from build123d import *

# Parameters (mm, degrees)
BOSS_EXTRUDE1_DEPTH = 6.35
SKETCH2_W           = 6.35
SKETCH2_H           = 1.5875
CUT_EXTRUDE1_DEPTH  = 6.35
BOSS_EXTRUDE2_START = -6.35
SKETCH4_W           = 24.326613467
SKETCH4_H           = 69.85
BOSS_EXTRUDE2_DEPTH = 6.35
SKETCH5_W           = 25.4
SKETCH5_H           = 3.175
CUT_EXTRUDE3_DEPTH  = 6.35
SKETCH7_W           = 19.923596682
SKETCH7_H           = 95.25
CUT_EXTRUDE4_DEPTH  = 6.35
SKETCH8_W           = 15.043251586
SKETCH8_H           = 69.85
CUT_EXTRUDE5_DEPTH  = 6.35
SKETCH9_W           = 3.175
SKETCH9_H           = 95.25
BOSS_EXTRUDE3_DEPTH = 6.35
SKETCH10_W          = 17.539756693
SKETCH10_H          = 95.25
CUT_EXTRUDE7_DEPTH  = 6.35
SKETCH3_W           = 4.7625
SKETCH3_H           = 14.2875
SKETCH3_W_2         = 9.525
SKETCH3_H_2         = 3.175
CUT_EXTRUDE8_DEPTH  = 6.35
SKETCH11_W          = 14.2875
SKETCH11_H          = 4.7625
SKETCH11_W_2        = 3.175
SKETCH11_H_2        = 7.9375
CUT_EXTRUDE9_DEPTH  = 6.35
SKETCH14_W          = 14.575398065
SKETCH14_H          = 32.31050226
CUT_EXTRUDE11_DEPTH = 6.35


with BuildPart() as part:
    # Sketch1 → Boss-Extrude1 (new body)
    with BuildSketch(Plane(origin=(0, 0, 0), x_dir=(1, 0, 0), z_dir=(0, 1, 0))):
        Polygon((38.1, 65.0875), (84.214756693, 65.0875), (84.214756693, -30.1625), (38.1, -30.1625), (38.1, -19.05), (19.05, -19.05), (19.05, -25.4), (6.35, -25.4), (6.35, -19.05), (0, -19.05), (0, 0), (0, 34.925), (0, 53.975), (6.35, 53.975), (6.35, 60.325), (19.05, 60.325), (19.05, 53.975), (38.1, 53.975), align=None)
        Polygon((38.1, 34.925), (44.45, 38.591174209), (44.45, 52.3875), (74.689756693, 52.3875), (77.864756693, 50.8), (77.864756693, -15.875), (74.689756693, -17.4625), (44.45, -17.4625), (44.45, -3.666174209), (38.1, 0), align=None, mode=Mode.SUBTRACT)
    extrude(amount=BOSS_EXTRUDE1_DEPTH)

    # Sketch2 → Cut-Extrude1 (cut)
    with BuildSketch(Plane(origin=(0, 6.35, 0), x_dir=(1, 0, 0), z_dir=(0, 1, 0))):
        with Locations((9.525, 35.71875)):
            Rectangle(SKETCH2_W, SKETCH2_H)
        with Locations((9.525, -0.79375)):
            Rectangle(SKETCH2_W, SKETCH2_H)
        with Locations((28.575, 35.71875)):
            Rectangle(SKETCH2_W, SKETCH2_H)
        with Locations((28.575, -0.79375)):
            Rectangle(SKETCH2_W, SKETCH2_H)
    extrude(amount=-CUT_EXTRUDE1_DEPTH, mode=Mode.SUBTRACT)

    # Sketch4 → Boss-Extrude2 (add)
    with BuildSketch(Plane(origin=(0, 6.35, 0), x_dir=(1, 0, 0), z_dir=(0, 1, 0)).offset(BOSS_EXTRUDE2_START)):
        with Locations((49.82644996, 17.4625)):
            Rectangle(SKETCH4_W, SKETCH4_H)
    extrude(amount=BOSS_EXTRUDE2_DEPTH)

    # Sketch5 → Cut-Extrude3 (cut)
    with BuildSketch(Plane(origin=(0, 6.35, 0), x_dir=(1, 0, 0), z_dir=(0, 1, 0))):
        with Locations((61.989756693, 17.4625)):
            Rectangle(SKETCH5_W, SKETCH5_H)
        with Locations((36.589756693, 17.4625)):
            Rectangle(SKETCH5_W, SKETCH5_H)
    extrude(amount=-CUT_EXTRUDE3_DEPTH, mode=Mode.SUBTRACT)

    # Sketch7 → Cut-Extrude4 (cut)
    with BuildSketch(Plane(origin=(0, 6.35, 0), x_dir=(1, 0, 0), z_dir=(0, 1, 0))):
        with Locations((91.001555034, 17.4625)):
            Rectangle(SKETCH7_W, SKETCH7_H)
    extrude(amount=-CUT_EXTRUDE4_DEPTH, mode=Mode.SUBTRACT)

    # Sketch8 → Cut-Extrude5 (cut)
    with BuildSketch(Plane.XZ):
        with Locations((52.803374207, -17.4625)):
            Rectangle(SKETCH8_W, SKETCH8_H)
    extrude(amount=-CUT_EXTRUDE5_DEPTH, mode=Mode.SUBTRACT)

    # Sketch9 → Boss-Extrude3 (add)
    with BuildSketch(Plane.XZ):
        with Locations((61.9125, -17.4625)):
            Rectangle(SKETCH9_W, SKETCH9_H)
    extrude(amount=-BOSS_EXTRUDE3_DEPTH)

    # Sketch10 → Cut-Extrude7 (cut)
    with BuildSketch(Plane.XZ):
        with Locations((72.269878347, -17.4625)):
            Rectangle(SKETCH10_W, SKETCH10_H)
    extrude(amount=-CUT_EXTRUDE7_DEPTH, mode=Mode.SUBTRACT)

    # Sketch3 → Cut-Extrude8 (cut)
    with BuildSketch(Plane(origin=(0, 6.35, 0), x_dir=(1, 0, 0), z_dir=(0, 1, 0))):
        with Locations((26.168267374, 46.83125)):
            Rectangle(SKETCH3_W, SKETCH3_H)
        with Locations((26.168267374, 44.45)):
            Rectangle(SKETCH3_W_2, SKETCH3_H_2)
        with Locations((26.168267374, -9.525)):
            Rectangle(SKETCH3_W_2, SKETCH3_H_2)
        with Locations((26.168267374, -11.90625)):
            Rectangle(SKETCH3_W, SKETCH3_H)
    extrude(amount=-CUT_EXTRUDE8_DEPTH, mode=Mode.SUBTRACT)

    # Sketch11 → Cut-Extrude9 (cut)
    with BuildSketch(Plane.XZ):
        with Locations((56.35625, 23.932056084)):
            Rectangle(SKETCH11_W, SKETCH11_H)
        with Locations((53.975, 23.932056084)):
            Rectangle(SKETCH11_W_2, SKETCH11_H_2)
        with Locations((53.975, -58.857056084)):
            Rectangle(SKETCH11_W_2, SKETCH11_H_2)
        with Locations((56.35625, -58.857056084)):
            Rectangle(SKETCH11_W, SKETCH11_H)
    extrude(amount=-CUT_EXTRUDE9_DEPTH, mode=Mode.SUBTRACT)

    # Sketch14 → Cut-Extrude11 (cut)
    with BuildSketch(Plane(origin=(0, 6.35, 0), x_dir=(1, 0, 0), z_dir=(0, 1, 0))):
        with Locations((67.612699033, -1.30724887)):
            Rectangle(SKETCH14_W, SKETCH14_H)
    extrude(amount=-CUT_EXTRUDE11_DEPTH, mode=Mode.SUBTRACT)


solid = part.part
The listing builds one solid part. Answer for the finished solid, in the listing's coordinates (mm). A direction names the side the tool comes from. Coordinates: 2 decimals unless noted, no trailing zeros. Write each loop counter-clockwise with the first axis right and the second up, starting at its lowest first coordinate (ties: lowest second). Pieces come first, ordered by that corner, then holes. Notation, with made-up numbers: (-17.5, 35.5) -> (30.5, 35.5) arc R23 ccw to (30.5, 51.5) -> close; hole circle Ø2 at (88, 73). An arc over 180 degrees is marked (long way). One line per question, with ' | ' between items.
1. Section B-B (z = -20.5) is taken. Determine the outline of the cut face in (x, y) (3 decimals), and give its area (3 significant figures).
Verdict:
outline: (0, 0) -> (45.282, 0) -> (45.282, 6.35) -> (0, 6.35) -> close; (60.325, 0) -> (63.5, 0) -> (63.5, 6.35) -> (60.325, 6.35) -> close | area: 308 mm^2
2. Given pin 1 Ø0.5 at (y, z) = (4.5, 20.5) entering from -X; pin 2 Ø0.5 at (y, z) = (3, 27) entering from -X, each flat-ended and moving along its own axis, determine where each tip first touches the part or whether it passes through.
Verdict:
pin 1: stops at x = 6.35 | pin 2: stops at x = 38.1
3. For a pull along Z with two mould halves and no side action, classify faces 1 (the flat face through (19.05, 3, -57)), 2 (the flat face through (51, 3, -65.088)), 3 (the flat face through (45.282, 3, 1)), 4 (the flat face through (49.213, 3, -59)) as released by +Z, released by -Z, zero draft, split by the parting line, or undercut.
Verdict:
face 1: zero draft | face 2: released by -Z | face 3: undercut | face 4: undercut
4. Which of the six approach directions +Z, -Z, +X, -X, +Y, -Y give full straight-line access (tool end or side, diameter ignored) to faces 5 (the flat face through (38.1, 3, 25)), 6 (the flat face through (6.35, 3, 22)), 7 (the flat face through (51, 3, 21.551)), 8 (the flat face through (30.931, 3, -44))?
Verdict:
face 5: +Z, +Y, -Y | face 6: +Z, -X, +Y, -Y | face 7: +X, +Y, -Y | face 8: +Y, -Y
5. Section A-A (x = 29.5) is taken. State how many separate pieces and enclosed holes the cut face has, and give its area (3 significant figures).
Verdict:
separate pieces: 6 | enclosed holes: 0 | area: 383 mm^2
6. Straight lines are drawn through the part: line 1 (X direction, y = 2.75, z = -35.5) (3 decimals); line 2 (X direction, y = 5.5, z = -47) (3 decimals); line 3 (Z direction, x = 12, y = 5.5) (1 decimal). For each, find the intervals that lie inside material, in ascending order.
Verdict:
line 1: x = 0 to 6.35, 12.7 to 25.4, 31.75 to 45.282, 60.325 to 63.5 | line 2: x = 0 to 23.787, 28.55 to 45.282, 60.325 to 63.5 | line 3: z = -60.3 to -36.5, -34.9 to 0, 1.6 to 25.4
